```python
from build123d import *

# Parameters (mm, degrees)
F0_W      = 52
F0_H      = 85
F1_DEPTH  = 20
F2_W      = 48
F2_H      = 83
F3_DEPTH  = 18
F5_DEPTH  = 5
F7_DEPTH  = 5
F8_W      = 1
F8_H      = 83
F9_DEPTH  = 3
F10_W     = 1
F10_H     = 83
F11_DEPTH = 3


with BuildPart() as f1:
    # F0 (on Top) → F1 (new body)
    with BuildSketch(Plane.XY):
        Rectangle(F0_W, F0_H)
    extrude(amount=F1_DEPTH)

    # F2 (on face) → F3 (cut)
    with BuildSketch(Plane.XY.offset(20)):
        Rectangle(F2_W, F2_H)
    extrude(amount=-F3_DEPTH, mode=Mode.SUBTRACT)

    # F4 (on face) → F5 (cut)
    with BuildSketch(Plane.XZ.offset(42.5)):
        Polygon((-20, 14), (0, 14), (20, 14), (20, 20), (-20, 20), align=None)
    extrude(amount=-F5_DEPTH, mode=Mode.SUBTRACT)

    # F6 (on face) → F7 (cut)
    with BuildSketch(Plane(origin=(0, 42.5, 0), x_dir=(-1, 0, 0), z_dir=(0, 1, 0))):
        with BuildLine():
            ThreePointArc((-9.2330926563, 20), (-5.3735463151, 15.9791907237), (0, 14.5))
            Line((0, 14.5), (0, 20))
            Line((0, 20), (-9.2330926563, 20))
        make_face()
        with BuildLine():
            Line((0, 20), (0, 14.5))
            ThreePointArc((0, 14.5), (5.3735463151, 15.9791907237), (9.2330926563, 20))
            Line((9.2330926563, 20), (0, 20))
        make_face()
    extrude(amount=-F7_DEPTH, mode=Mode.SUBTRACT)

    # F8 (on face) → F9 (cut)
    with BuildSketch(Plane.XY.offset(20)):
        with Locations((24.5, 0)):
            Rectangle(F8_W, F8_H)
    extrude(amount=-F9_DEPTH, mode=Mode.SUBTRACT)

    # F10 (on face) → F11 (cut)
    with BuildSketch(Plane.XY.offset(20)):
        with Locations((-24.5, 0)):
            Rectangle(F10_W, F10_H)
    extrude(amount=-F11_DEPTH, mode=Mode.SUBTRACT)


solid = f1.part
```
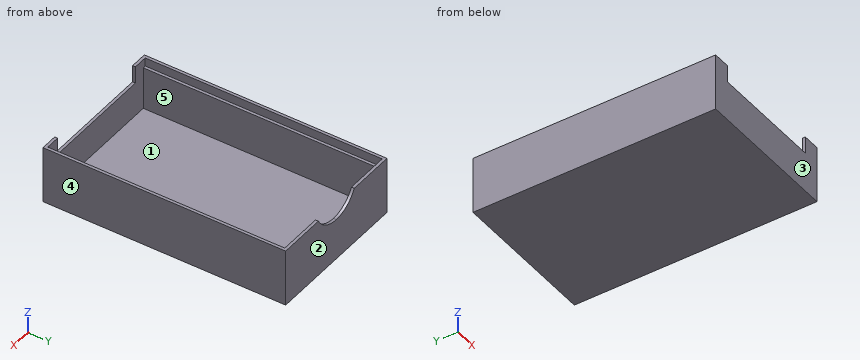
Design review of the part built by this model. Coordinates are the model's own, in mm. Face numbers are marked on the shaded views. A direction names the side the tool comes from. Round coordinates to 2 decimals unless told otherwise and drop trailing zeros. Write each loop counter-clockwise with the first axis right and the second up, starting at its lowest first coordinate (ties: lowest second). Pieces come first, ordered by that corner, then holes. Notation, with made-up numbers: (-11, 46) -> (7, 46) arc R17 ccw to (7, 62) -> close; hole circle Ø4 at (45.5, 73). An arc over 180 degrees is marked (long way). Write item = value, one per line. Start each with the question number.
1) Wall thickness on probe 1 along Y at (x, z) = (-3, 11); probe 2 along X at (y, z) = (-20.5, 9.5); probe 3 along X at (y, z) = (-35.5, 19): over which ranges is each line inside the solid? List them lowest first. Write a range as from..to.
2) Take a section at C-C, the plane y = 27. State the section outline as (x, z) points, plus the area to 3 significant figures.
3) Take a section at A-A, the plane z = 15.5. State the section outline as (x, y) points.
4) Tool access review of the marked faces 4 and 5: name each direction out of +Z, -Z, +X, -X, +Y, -Y from which nothing blocks a thin tool from reaching the whole face with its end or side.
5) Mouldability with a two-part tool opening along Y and no side actions: class the marked faces 1, 2 and 3 as +Y half, -Y half, draft (parallel to the pull), parting line (faces both ways), or undercut.
6) Take a section at D-D, the plane x = -23. State the section outline as (y, z) points.
7) Take a section at B-B, the plane x = -13. State the section outline as (y, z) points, plus the area to 3 significant figures.
8) Clearance check with flat-ended pins moving along their axes: pin 1 (0.8 mm diameter, centred on x = 6, y = -42, fed in from +Z); pin 2 (0.8 mm diameter, centred on x = 24.5, y = -8.5, fed in from +Z); pin 3 (3 mm diameter, centred on x = -16, z = 17, fed in from -Y). State where each tip first meets the part, or that it passes through.
Results list:
q1.probe_1 = -42.5..-41.5, 41.5..42.5
q1.probe_2 = -26..-24, 24..26
q1.probe_3 = -26..-25, 25..26
q2.outline = (-26, 0) -> (26, 0) -> (26, 20) -> (25, 20) -> (25, 17) -> (24, 17) -> (24, 2) -> (-24, 2) -> (-24, 17) -> (-25, 17) -> (-25, 20) -> (-26, 20) -> close
q2.area = 170 mm²
q3.outline = (-26, -42.5) -> (-20, -42.5) -> (-20, -41.5) -> (-24, -41.5) -> (-24, 41.5) -> (-4.47, 41.5) -> (-4.47, 42.5) -> (-26, 42.5) -> close; (4.47, 41.5) -> (24, 41.5) -> (24, -41.5) -> (20, -41.5) -> (20, -42.5) -> (26, -42.5) -> (26, 42.5) -> (4.47, 42.5) -> close
q4.face_4 = +Z, -Z, +X, +Y, -Y
q4.face_5 = +Z
q5.face_1 = undercut
q5.face_2 = +Y half
q5.face_3 = -Y half
q6.outline = (-42.5, 0) -> (42.5, 0) -> (42.5, 20) -> (41.5, 20) -> (41.5, 2) -> (-41.5, 2) -> (-41.5, 20) -> (-42.5, 20) -> close
q7.outline = (-42.5, 0) -> (42.5, 0) -> (42.5, 20) -> (41.5, 20) -> (41.5, 2) -> (-41.5, 2) -> (-41.5, 14) -> (-42.5, 14) -> close
q7.area = 200 mm²
q8.pin_1 = 14
q8.pin_2 = 17
q8.pin_3 = 41.5
